from build123d import *

# Parameters (mm, degrees)
F0_R     = 57.15
F1_DEPTH = 14.224
F2_R     = 15.875
F3_DEPTH = 14.225
F4_R     = 7.112
F5_DEPTH = 14.225
F7_DEPTH = 30.226


with BuildPart() as f1:
    # F0 (on Front) → F1 (new body)
    with BuildSketch(Plane.XZ):
        Circle(F0_R)
    extrude(amount=F1_DEPTH)

    # F2 (on face) → F3 (cut, through all)
    with BuildSketch(Plane.XZ.offset(14.224)):
        Circle(F2_R)
    extrude(amount=-F3_DEPTH, mode=Mode.SUBTRACT)

    # F4 (on face) → F5 (cut, through all)
    with BuildSketch(Plane.XZ.offset(14.224)):
        with Locations((0, -36.576)):
            Circle(F4_R)
        with Locations((31.675745, 18.288)):
            Circle(F4_R)
        with Locations((-31.675745, 18.288)):
            Circle(F4_R)
    extrude(amount=-F5_DEPTH, mode=Mode.SUBTRACT)

    # F6 (on face) → F7 (join)
    with BuildSketch(Plane.XZ.offset(14.224)):
        with BuildLine():
            ThreePointArc((-18.485466, -33.315125), (-32.832196, -19.330206), (-38.1, 0))
            Line((-38.1, 0), (-50.8, 0))
            ThreePointArc((-50.8, 0), (-43.886307, -25.585779), (-25.027083, -44.207297))
            Line((-25.027083, -44.207297), (-18.485466, -33.315125))
        make_face()
        with BuildLine():
            Line((50.8, 0), (38.1, 0))
            ThreePointArc((38.1, 0), (32.493945, -19.893555), (17.325537, -33.932813))
            Line((17.325537, -33.932812), (23.487626, -45.044105))
            ThreePointArc((23.487626, -45.044105), (43.438528, -26.338836), (50.8, 0))
        make_face()
        with BuildLine():
            Line((20.723909, 31.970762), (27.265526, 42.862934))
            ThreePointArc((27.265526, 42.862934), (0.876096, 50.792445), (-25.771101, 43.777738))
            Line((-25.771101, 43.777738), (-19.609012, 32.666446))
            ThreePointArc((-19.609012, 32.666446), (0.657072, 38.094334), (20.723909, 31.970762))
        make_face()
    extrude(amount=F7_DEPTH)


solid = f1.part
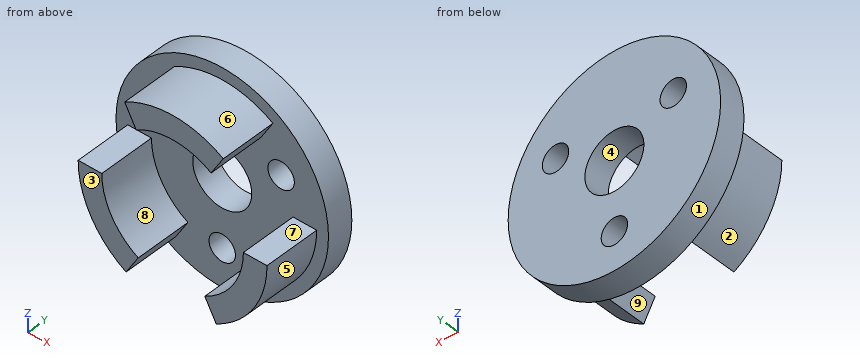
Design review of the part built by this model. Coordinates are the model's own, in mm. Face numbers are marked on the shaded views. A direction names the side the tool comes from. Give positions to 0.01 mm unless a question says otherwise; leave off trailing zeros. Write each loop counter-clockwise with the first axis right and the second up, starting at its lowest first coordinate (ties: lowest second). Pieces come first, ordered by that corner, then holes. Notation, with made-up numbers: M -5.75,-20 L 47.25,-20 A24 ccw 47.25,13 Z; hole C 79,6.25 d6. An arc over 180 degrees is marked long. Return JSON: item names as keys, results as strings. Group by question number.
Item 1: Tool access review of the marked faces 5, 6, 7, 8 and 9: name each direction out of +Z, -Z, +X, -X, +Y, -Y from which nothing blocks a thin tool from reaching the whole face with its end or side.
Item 2: Wall thickness on line 1 along Z through (x, y) = (0, -7) (3 decimals); line 2 along Y through (x, z) = (-41, 12); line 3 along X through (y, z) = (-2.5, 21): over which ranges is each line inside the solid? List them lowest first.
Item 3: The part is to be moulded in two halves that separate along X. For the marked faces 1, 2, 3 and 4, say which applies: pulls with the +X half, pulls with the -X half, needs draft (parallel to the pull), parting line crosses it, or undercut.
Item 4: Take a section at B-B (y = -25). Give the boundary of the cut face in (x, z).
Item 5: Take a section at A-A (x = 0). Give the boundary of the cut face in (y, z) (3 decimals).
Item 6: Take a section at D-D (x = -29.5). Give the boundary of the cut face in (y, z), plus the area to 3 significant figures.
Item 7: Take a section at C-C (z = -41.5). Give the boundary of the cut face in (x, y), plus the area to 3 significant figures.
Item 8: Clearance check with flat-ended pins moving along their axes: pin 1 Ø1.5 at (y, z) = (-31, -15.5) entering from -X; pin 2 Ø1 at (y, z) = (-38, -30.5) entering from +X; pin 3 Ø18.5 at (x, z) = (-31.68, 18.29) entering from -Y. State where each tip first meets the part, or that it passes through.
Return value:
{
 "1": {"face 5": "-Z, +X, -Y", "face 6": "+Z, -Y", "face 7": "+Z, +X, -X, -Y", "face 8": "-Y", "face 9": "-Z, -Y"},
 "2": {"line 1": "z = -57.15 to -43.688, -29.464 to -15.875, 15.875 to 57.15", "line 2": "y = -14.22 to 0", "line 3": "x = -53.15 to -38.25, -25.1 to 25.1, 38.25 to 53.15"},
 "3": {"face 1": "parting line crosses it", "face 2": "pulls with the -X half", "face 3": "needs draft", "face 4": "undercut"},
 "4": {"outline": "M -50.8,0 A50.8 ccw -25.03,-44.21 L -18.49,-33.32 A38.1 cw -38.1,0 Z; M -25.77,43.78 L -19.61,32.67 A38.1 cw 20.72,31.97 L 27.27,42.86 A50.8 ccw Z; M 17.33,-33.93 L 23.49,-45.04 A50.8 ccw 50.8,0 L 38.1,0 A38.1 cw Z"},
 "5": {"outline": "M -44.45,38.1 L -14.224,38.1 L -14.224,15.875 L 0,15.875 L 0,57.15 L -14.224,57.15 L -14.224,50.8 L -44.45,50.8 Z; M -14.224,-57.15 L 0,-57.15 L 0,-43.688 L -14.224,-43.688 Z; M -14.224,-29.464 L 0,-29.464 L 0,-15.875 L -14.224,-15.875 Z"},
 "6": {"outline": "M -44.45,-41.36 L -14.22,-41.36 L -14.22,-48.95 L 0,-48.95 L 0,11.52 L -14.22,11.52 L -14.22,-24.11 L -44.45,-24.11 Z; M -14.22,25.06 L 0,25.06 L 0,48.95 L -14.22,48.95 Z", "area": "1,720 mm2"},
 "7": {"outline": "M -39.29,-14.22 L -29.3,-14.22 L -29.3,-44.45 L -23.4,-44.45 L -23.4,-14.22 L -5.13,-14.22 L -5.13,0 L -39.29,0 Z; M 5.13,-14.22 L 21.52,-14.22 L 21.52,-44.45 L 29.3,-44.45 L 29.3,-14.22 L 39.29,-14.22 L 39.29,0 L 5.13,0 Z", "area": "1,390 mm2"},
 "8": {"pin 1": "stops at x = -48.61", "pin 2": "stops at x = 41", "pin 3": "stops at y = -14.22"}
}
